from build123d import *

# Parameters (mm, degrees)
SKETCH1_W           = 22.8
SKETCH1_H           = 12.7
BODY_DEPTH          = 22
SKETCH2_W           = 4.6
SKETCH2_H           = 12.7
SKETCH2_R           = 1.125
BOSS_EXTRUDE2_DEPTH = 2.3
SKETCH3_R           = 2.35
BOSS_EXTRUDE3_DEPTH = 7.2
SKETCH4_R           = 6.35
BOSS_EXTRUDE4_DEPTH = 4.25


with BuildPart() as part:
    # Sketch1 → Body (new body)
    with BuildSketch(Plane.XY):
        Rectangle(SKETCH1_W, SKETCH1_H)
    extrude(amount=BODY_DEPTH)

    # Sketch2 → Boss-Extrude2 (add)
    with BuildSketch(Plane(origin=(0, 0, 16), x_dir=(-1, 0, 0), z_dir=(0, 0, -1))):
        with Locations((13.7, 0)):
            Rectangle(SKETCH2_W, SKETCH2_H)
        with Locations((13.7, 0)):
            Circle(SKETCH2_R, mode=Mode.SUBTRACT)
        with Locations((-13.7, 0)):
            Rectangle(SKETCH2_W, SKETCH2_H)
        with Locations((-13.7, 0)):
            Circle(SKETCH2_R, mode=Mode.SUBTRACT)
    extrude(amount=-BOSS_EXTRUDE2_DEPTH)

    # Sketch3 → Boss-Extrude3 (add)
    with BuildSketch(Plane.XY.offset(22)):
        with Locations((5.05, 0)):
            Circle(SKETCH3_R)
    extrude(amount=BOSS_EXTRUDE3_DEPTH)

    # Sketch4 → Boss-Extrude4 (add)
    with BuildSketch(Plane.XY.offset(22)):
        with Locations((5.05, 0)):
            Circle(SKETCH4_R)
    extrude(amount=BOSS_EXTRUDE4_DEPTH)


solid = part.part
Here's how the part is built. I have some questions about the finished solid (model axes, mm). A direction names the side the tool comes from. Round coordinates to 2 decimals unless told otherwise and drop trailing zeros. Write each loop counter-clockwise with the first axis right and the second up, starting at its lowest first coordinate (ties: lowest second). Pieces come first, ordered by that corner, then holes.
1. Suppose I cut it at A-A (x = -13.7). List the corners of the cut face in (y, z) for me (3 decimals), and give its area (3 significant figures).
2. For faces 1 (the flat face through (13.7, -1.3, 16)), 2 (the flat face through (-11.4, 0, 20)), 3 (the flat face through (5, -3, 26.25)), which set-ups out of +Z, -Z, +X, -X, +Y, -Y let a thin tool reach every point of the face, with its end or its side?
3. Will these pins go through, and if not, where does the flat tip stop? pin 1 Ø2.5 at (x, y) = (13.5, 2) entering from +Z; pin 2 Ø4 at (y, z) = (2, 21) entering from -X; pin 3 Ø2 at (x, y) = (-10.5, 4) entering from +Z; pin 4 Ø2 at (x, y) = (-13.7, 0) entering from -Z.
4. Suppose I cut it at B-B (y = 3.75). List the corners of the cut face in (x, z) for me, and give its area (3 significant figures).
5. Suppose I cut it at C-C (x = 11). List the corners of the cut face in (y, z) for me.
6. If we mould it in two halves opening along Y, with no side actions, what happens to faces 4 (the flat face through (0, 6.35, 11)), 5 (the flat face through (16, 0, 17)), 6 (the flat face through (0, -6.35, 11)), 7 (the cylindrical face through (12.627, 0.338, 17.134))? For each: released by +Y, released by -Y, zero draft, split by the parting line, or undercut.
7. I need wall thicknesses on L1, parallel to Y at x = 13.7, z = 16.65 (3 decimals); L2, parallel to Z at x = 3, y = 4.75; L3, parallel to Z at x = -2, y = -1. Which ranges of each line are inside material? Lowest first, please.
8. Suppose I cut it at D-D (z = 12.25). List the corners of the cut face in (x, y) for me, and give its area (3 significant figures).
Answer sheet:
1. outline: (-6.35, 16) - (-1.125, 16) - (-1.125, 18.3) - (-6.35, 18.3) - close; (1.125, 16) - (6.35, 16) - (6.35, 18.3) - (1.125, 18.3) - close
1. area: 24.0 mm2
2. face 1: -Z, +X, +Y, -Y
2. face 2: +Z, -X, +Y, -Y
2. face 3: +Z
3. pin 1: stops at z = 18.3
3. pin 2: stops at x = -11.4
3. pin 3: stops at z = 22
3. pin 4: passes through
4. outline: (-16, 16) - (-11.4, 16) - (-11.4, 0) - (11.4, 0) - (11.4, 16) - (16, 16) - (16, 18.3) - (11.4, 18.3) - (11.4, 22) - (10.17, 22) - (10.17, 26.25) - (-0.07, 26.25) - (-0.07, 22) - (-11.4, 22) - (-11.4, 18.3) - (-16, 18.3) - close
4. area: 566 mm2
5. outline: (-6.35, 0) - (6.35, 0) - (6.35, 22) - (2.22, 22) - (2.22, 26.25) - (-2.22, 26.25) - (-2.22, 22) - (-6.35, 22) - close
6. face 4: released by +Y
6. face 5: zero draft
6. face 6: released by -Y
6. face 7: undercut
7. L1: y = -6.35 to -1.125, 1.125 to 6.35
7. L2: z = 0 to 26.25
7. L3: z = 0 to 22
8. outline: (-11.4, -6.35) - (11.4, -6.35) - (11.4, 6.35) - (-11.4, 6.35) - close
8. area: 290 mm2
